Part model, mm, in its own coordinate system. A direction names the side the tool comes from. Round coordinates to 2 decimals unless told otherwise and drop trailing zeros. Write each loop counter-clockwise with the first axis right and the second up, starting at its lowest first coordinate (ties: lowest second). Pieces come first, ordered by that corner, then holes. Notation, with made-up numbers: (-28, 80) -> (27, 80) arc R18 ccw to (27, 91) -> close; hole circle Ø3 at (70.25, 79.25). An arc over 180 degrees is marked (long way). Return JSON: item names as keys, results as strings. Group by question number.
```python
from build123d import *

# Parameters (mm, degrees)
F1_DEPTH = 63.5
F0_W     = 25.4
F0_H     = 19.05
F2_DEPTH = 25.4
F3_DEPTH = 7.9375
F5_R     = 6.35
F6_SIZE  = 1.5875


with BuildPart() as f1:
    # F0 (on Front) → F1 (new body, symmetric)
    with BuildSketch(Plane.XZ):
        Polygon((-41.275, -9.525), (41.275, -9.525), (41.275, 9.525), (22.225, 9.525), (-41.275, 9.525), align=None)
    extrude(amount=F1_DEPTH, both=True)

    # F0 (on Front) → F2 (join, symmetric)
    with BuildSketch(Plane.XZ):
        with BuildLine():
            Line((22.225, 9.525), (41.275, 9.525))
            Line((41.275, 9.525), (41.275, 27.0018676308))
            ThreePointArc((41.275, 27.0018676308), (46.1660118217, 38.4634394558), (57.8252524344, 42.8625))
            Line((57.8252524344, 42.8625), (60.325, 42.8625))
            Line((60.325, 42.8625), (60.325, 61.9125))
            Line((60.325, 61.9125), (58.151684873, 61.9125))
            ThreePointArc((58.151684873, 61.9125), (32.8110211717, 52.0492174826), (22.225, 27.0018676308))
            Line((22.225, 27.0018676308), (22.225, 9.525))
        make_face()
        with Locations((73.025, 52.3875)):
            Rectangle(F0_W, F0_H)
    extrude(amount=F2_DEPTH, both=True)

    # F0 (on Front) → F3 (join, symmetric)
    with BuildSketch(Plane.XZ):
        with BuildLine():
            add(Edge.make_bspline(
                [(-41.275, 9.525), (-42.120564729, 35.0021496415), (12.7173494548, 67.8302869201), (58.151684873, 61.9125)],
                knots=[0, 0, 0, 0, 112.3837880706, 112.3837880706, 112.3837880706, 112.3837880706], degree=3))
            Line((-41.275, 9.525), (22.225, 9.525))
            Line((22.225, 9.525), (22.225, 27.0018676308))
            ThreePointArc((22.225, 27.0018676308), (32.8110211717, 52.0492174826), (58.151684873, 61.9125))
        make_face()
    extrude(amount=F3_DEPTH, both=True)

    # F0 (on Front) → F4 (revolve)
    with BuildSketch(Plane.XZ):
        Polygon((85.725, 66.675), (85.725, 61.9125), (85.725, 42.8625), (85.725, 38.1), (111.125, 38.1), (111.125, 66.675), align=None)
    revolve(axis=Axis((85.725, 0, 52.3875), (0, 0, -1)))

    # F5
    f5_edges = [f1.edges().sort_by_distance(p)[0] for p in [
        (41.275, -63.5, 0),
        (41.275, 63.5, 0),
        (-41.275, -63.5, 0),
        (-41.275, 63.5, 0),
    ]]
    fillet(f5_edges, radius=F5_R)

    # F6
    f6_edges = [f1.edges().sort_by_distance(p)[0] for p in [
        (60.325, 0, 66.675),
        (60.325, 0, 38.1),
    ]]
    chamfer(f6_edges, length=F6_SIZE)


solid = f1.part
```
Item 1: Which spindle directions (+Z, -Z, +X, -X, +Y, -Y) get a long thin tool onto all of the face, cutting with end or side? Do faces 1 (the face through (41.275, -1, 4)), 2 (the face through (-41.275, -1, 0)), 3 (the face through (-2, -7.938, 33)), 4 (the face through (22.225, 17, 18)), 5 (the face through (46, -25.4, 42)). Say none if no direction does.
Item 2: Wall check: L1, parallel to Z at x = -28.5, y = 8 (3 decimals); L2, parallel to Y at x = 32.5, z = 26; L3, parallel to X at y = -42.5, z = 3 (3 decimals). Give the ranges that are in metal, low to high.
Item 3: Cut at A-A (y = -33). Write the cut outline in (x, z) (3 decimals), then the cut area to 3 significant figures.
Item 4: Flat gauge pins, fed straight in: P1, Ø2, axis at x = -7.5, y = 2.5, coming from the +Z side; P2, Ø21, axis at y = 10.5, z = 0.5, coming from the -X side; P3, Ø5, axis at y = 18.5, z = 16.5, coming from the -X side (3 decimals); P4, Ø16, axis at x = 12.5, z = 37.5, coming from the +Y side. Where does each tip first touch, or does it go through?
Checks:
{
 "1": {"face 1": "-Z, +X, +Y, -Y", "face 2": "+Z, -Z, -X, +Y, -Y", "face 3": "+Z, -X, -Y", "face 4": "+Z, -X, +Y", "face 5": "+Z, +X, -X, -Y"},
 "2": {"L1": "z = -9.525 to 9.525", "L2": "y = -25.4 to 25.4", "L3": "x = -41.275 to 41.275"},
 "3": {"outline": "(-41.275, -9.525) -> (41.275, -9.525) -> (41.275, 9.525) -> (-41.275, 9.525) -> close", "area": "1,570 mm2"},
 "4": {"P1": "stops at z = 48.79", "P2": "stops at x = -41.28", "P3": "stops at x = 22.225", "P4": "stops at y = 7.94"}
}
